Verification items for the finished model (mm, model axes). A direction names the side the tool comes from. Round coordinates to 2 decimals unless told otherwise and drop trailing zeros. Write each loop counter-clockwise with the first axis right and the second up, starting at its lowest first coordinate (ties: lowest second). Pieces come first, ordered by that corner, then holes. Notation, with made-up numbers: M 4,4.25 L 9,4.25 A35 ccw 9,38.25 Z; hole C -37.75,10.25 d8. An arc over 180 degrees is marked long. Answer in a Markdown table with one row per item. Add a question column.
1. Sectioned sample at B-B on y = 0.75. Count the separate pieces of the cut face and the enclosed holes in it, plus the area to 3 significant figures.
2. Sectioned sample at C-C on z = -8.5. Record the cut outline in (x, y).
3. Sectioned sample at A-A on x = -63. Record the cut outline in (y, z), plus the area to 3 significant figures.
4. Draft check along Z on faces 1 (the flat face through (-65, 1, -31.508)), 2 (the flat face through (-96.25, 0.99, 14.46)), 3 (the cylindrical face through (-78.9, 0.99, -25.95)). Enter one of: pulls with the +Z half, pulls with the -Z half, needs draft (parallel to the pull), parting line crosses it, or undercut.
5. Go/stop test with flat-tipped pins: pin 1 Ø0.6 at (x, y) = (-65, 1) entering from +Z; pin 2 Ø1 at (x, y) = (-64.5, 1) entering from -Z; pin 3 Ø1 at (y, z) = (1, 10.5) entering from -X. Record where each tip stops, or that it passes through.
6. Material ranges on probe 1 along Z at (x, y) = (-39, 0.15); probe 2 along Z at (x, y) = (-36, 0.3); probe 3 along X at (y, z) = (1.05, -1), recorded low to high.
7. Set-up check for faces 4 (the flat face through (-98.057, 0.986, -19.029)), 5 (the cylindrical face through (-52.513, 0.986, -33.073)), 6 (the flat face through (-44.384, 0.986, 16.092)), 7 (the flat face through (-32.81, 0.99, 7.97)), 8 (the cylindrical face through (-78.676, 0.986, 3.546)): record each of +Z, -Z, +X, -X, +Y, -Y from which the full face is reachable in a straight line by a thin tool's end or side.
```python
from build123d import *

# Parameters (mm, degrees)
SKETCH1_R           = 1.5
BOSS_EXTRUDE1_DEPTH = 2


with BuildPart() as part:
    # Sketch1 → Boss-Extrude1 (new body)
    # profile 1 of 5: a face of its own
    with BuildSketch(Plane(origin=(0, 0, 0), x_dir=(1, 0, 0), z_dir=(0, 1, 0))):
        with BuildLine():
            Line((-46.126205575, -14.349426059), (-42.591934327, -17.883697307))
            ThreePointArc((-42.591934327, -17.883697307), (-37.566674414, -19.121078278), (-34.137468144, -15.244882561))
            Line((-34.137468144, -15.244882561), (-31.447944327, -0.491561683))
            Line((-31.447944327, -0.491561683), (-31.447944327, 23.508438317))
            Line((-31.447944327, 23.508438317), (-34.137468144, 38.261759196))
            ThreePointArc((-34.137468144, 38.261759196), (-37.566674414, 42.137954912), (-42.591934327, 40.900573941))
            Line((-42.591934327, 40.900573941), (-46.126205575, 37.366302693))
            ThreePointArc((-46.126205575, 37.366302693), (-52.614672551, 33.030847667), (-60.268341199, 31.508438317))
            Line((-60.268341199, 31.508438317), (-69.55766308, 31.508438317))
            ThreePointArc((-69.55766308, 31.508438317), (-77.211331727, 33.030847667), (-83.699798704, 37.366302693))
            Line((-83.699798704, 37.366302693), (-87.234069951, 40.900573941))
            ThreePointArc((-87.234069951, 40.900573941), (-92.450628543, 42.073984291), (-95.744809303, 37.862363639))
            Line((-95.744809303, 37.862363639), (-97.179633644, 23.508438317))
            Line((-97.179633644, 23.508438317), (-97.179633644, -0.491561683))
            Line((-97.179633644, -0.491561683), (-95.744809303, -14.845487005))
            ThreePointArc((-95.744809303, -14.845487005), (-92.450628543, -19.057107657), (-87.234069951, -17.883697307))
            Line((-87.234069951, -17.883697307), (-83.699798704, -14.349426059))
            ThreePointArc((-83.699798704, -14.349426059), (-77.211331727, -10.013971033), (-69.55766308, -8.491561683))
            Line((-69.55766308, -8.491561683), (-60.268341199, -8.491561683))
            ThreePointArc((-60.268341199, -8.491561683), (-52.614672551, -10.013971033), (-46.126205575, -14.349426059))
        make_face()
        with Locations(Location((-39.056400421, -14.348163401, 0), (0, 0, 270))):
            Circle(SKETCH1_R, mode=Mode.SUBTRACT)
        with Locations(Location((-39.056400421, 37.365040035, 0), (0, 0, 270))):
            Circle(SKETCH1_R, mode=Mode.SUBTRACT)
        with Locations(Location((-90.769603857, -14.348163401, 0), (0, 0, 270))):
            Circle(SKETCH1_R, mode=Mode.SUBTRACT)
        with Locations(Location((-49.663002139, -3.741561683, 0), (0, 0, 270))):
            Circle(SKETCH1_R, mode=Mode.SUBTRACT)
        with Locations(Location((-80.163002139, -3.741561683, 0), (0, 0, 270))):
            Circle(SKETCH1_R, mode=Mode.SUBTRACT)
        with Locations(Location((-80.163002139, 26.758438317, 0), (0, 0, 270))):
            Circle(SKETCH1_R, mode=Mode.SUBTRACT)
        with Locations(Location((-49.663002139, 26.758438317, 0), (0, 0, 270))):
            Circle(SKETCH1_R, mode=Mode.SUBTRACT)
        with Locations(Location((-36.913002139, 22.508438317, 0), (0, 0, 270))):
            Circle(SKETCH1_R, mode=Mode.SUBTRACT)
        with Locations(Location((-36.913002139, 0.508438317, 0), (0, 0, 270))):
            Circle(SKETCH1_R, mode=Mode.SUBTRACT)
        with Locations(Location((-92.913002139, 0.508438317, 0), (0, 0, 270))):
            Circle(SKETCH1_R, mode=Mode.SUBTRACT)
        with Locations(Location((-92.913002139, 22.508438317, 0), (0, 0, 270))):
            Circle(SKETCH1_R, mode=Mode.SUBTRACT)
        with Locations(Location((-90.769603857, 37.365040035, 0), (0, 0, 270))):
            Circle(SKETCH1_R, mode=Mode.SUBTRACT)
    # profile 2 of 5: a face of its own
    with BuildSketch(Plane(origin=(0, 0, 0), x_dir=(1, 0, 0), z_dir=(0, 1, 0))):
        with BuildLine():
            Line((-95.744809303, -14.845487005), (-97.179633644, -0.491561683))
            Line((-97.179633644, -0.491561683), (-97.179633644, -9.491561683))
            Line((-97.179633644, -9.491561683), (-97.179633644, -12.491561683))
            Line((-97.179633644, -12.491561683), (-95.289163865, -16.486755774))
            ThreePointArc((-95.289163865, -16.486755774), (-95.5873921, -15.685667214), (-95.744809303, -14.845487005))
        make_face()
    # profile 3 of 5: a face of its own
    with BuildSketch(Plane(origin=(0, 0, 0), x_dir=(1, 0, 0), z_dir=(0, 1, 0))):
        with BuildLine():
            Line((-97.179633644, 23.508438317), (-95.744809303, 37.862363639))
            ThreePointArc((-95.744809303, 37.862363639), (-95.5873921, 38.702543848), (-95.289163865, 39.503632408))
            Line((-95.289163865, 39.503632408), (-97.179633644, 35.508438317))
            Line((-97.179633644, 35.508438317), (-97.179633644, 32.508438317))
            Line((-97.179633644, 32.508438317), (-97.179633644, 23.508438317))
        make_face()
    # profile 4 of 5: a face of its own
    with BuildSketch(Plane(origin=(0, 0, 0), x_dir=(1, 0, 0), z_dir=(0, 1, 0))):
        Polygon((-97.179633644, 17.508438317), (-97.179633644, 23.508438317), (-97.179633644, 32.508438317), (-98.909633644, 28.508438317), (-98.909633644, 20.508438317), align=None)
    # profile 5 of 5: a face of its own
    with BuildSketch(Plane(origin=(0, 0, 0), x_dir=(1, 0, 0), z_dir=(0, 1, 0))):
        Polygon((-97.179633644, -0.491561683), (-97.179633644, 5.508438317), (-98.909633644, 2.508438317), (-98.909633644, -5.491561683), (-97.179633644, -9.491561683), align=None)
    extrude(amount=BOSS_EXTRUDE1_DEPTH)


solid = part.part
```
Geometry check:
| question | item | result |
|---|---|---|
| 1 | separate pieces | 1 |
| 1 | enclosed holes | 12 |
| 1 | area | 3,150 mm2 |
| 2 | outline | M -97.18,0 L -31.45,0 L -31.45,2 L -97.18,2 Z |
| 3 | outline | M 0,-31.51 L 2,-31.51 L 2,8.49 L 0,8.49 Z |
| 3 | area | 80.0 mm2 |
| 4 | face 1 | pulls with the -Z half |
| 4 | face 2 | pulls with the +Z half |
| 4 | face 3 | undercut |
| 5 | pin 1 | stops at z = 8.49 |
| 5 | pin 2 | stops at z = -31.51 |
| 5 | pin 3 | stops at x = -97.18 |
| 6 | probe 1 | z = -42.36 to -38.86, -35.87 to 12.85, 15.85 to 19.35 |
| 6 | probe 2 | z = -41.32 to -23.7, -21.32 to -1.7, 0.68 to 18.31 |
| 6 | probe 3 | x = -98.91 to -94.33, -91.5 to -38.33, -35.5 to -31.45 |
| 7 | face 4 | -X, +Y, -Y |
| 7 | face 5 | -Z, +Y, -Y |
| 7 | face 6 | +Z, +Y, -Y |
| 7 | face 7 | +Z, +X, +Y, -Y |
| 7 | face 8 | +Y, -Y |
